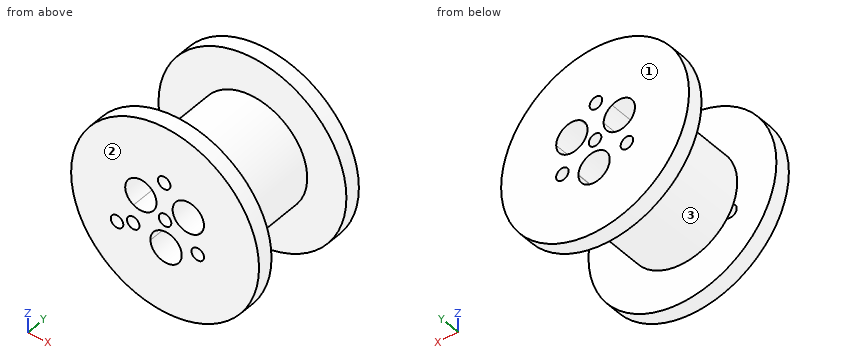
```python
from build123d import *

# Parameters (mm, degrees)
SKETCH1_R           = 30
BOSS_EXTRUDE1_DEPTH = 40
CUT_EXTRUDE1_START  = -5
SKETCH2_OUTSIDE_W   = 80.762
SKETCH2_OUTSIDE_H   = 80.762
SKETCH2_OUTSIDE_R   = 17.5
CUT_EXTRUDE1_DEPTH  = 30
SKETCH3_R           = 2
CUT_EXTRUDE2_DEPTH  = 59.309518948
CUT_EXTRUDE3_DEPTH  = 59.309518948
CUT_EXTRUDE4_REACH  = 57
SKETCH5_R           = 2
SKETCH8_R           = 2
CUT_EXTRUDE5_DEPTH  = 59.309518948


with BuildPart() as part:
    # Sketch1 → Boss-Extrude1 (new body)
    with BuildSketch(Plane(origin=(0, 0, 0), x_dir=(1, 0, 0), z_dir=(0, 1, 0))):
        with Locations(Location((0, 0, 0), (0, 0, 270))):
            Circle(SKETCH1_R)
    extrude(amount=BOSS_EXTRUDE1_DEPTH)

    # Sketch2 outside → Cut-Extrude1 (cut)
    with BuildSketch(Plane.XZ.offset(CUT_EXTRUDE1_START)):
        Rectangle(SKETCH2_OUTSIDE_W, SKETCH2_OUTSIDE_H)
        with Locations(Location((0, 0, 0), (0, 0, 270))):
            Circle(SKETCH2_OUTSIDE_R, mode=Mode.SUBTRACT)
    extrude(amount=-CUT_EXTRUDE1_DEPTH, mode=Mode.SUBTRACT)

    # Sketch3 → Cut-Extrude2 (cut, through all)
    with BuildSketch(Plane.XZ):
        with Locations(Location((0, 0, 0), (0, 0, 270))):
            Circle(SKETCH3_R)
    extrude(amount=-CUT_EXTRUDE2_DEPTH, mode=Mode.SUBTRACT)

    # Sketch4 → Cut-Extrude3 (cut, through all)
    with BuildSketch(Plane.XZ):
        with BuildLine():
            ThreePointArc((5.314601624, -8.562564428), (0.136244015, -3.747524192), (-4.678796221, -8.925881801))
            Line((-4.678796221, -8.925881801), (5.314601624, -8.562564428))
        make_face()
        with BuildLine():
            Line((5.314601624, -8.562564428), (-4.678796221, -8.925881801))
            ThreePointArc((-4.678796221, -8.925881801), (0.40874704, -13.743397777), (5.317902702, -8.744223114))
            ThreePointArc((5.317902702, -8.744223114), (5.317077364, -8.653378776), (5.314601624, -8.562564428))
        make_face()
        with BuildLine():
            ThreePointArc((4.758097504, 8.883862231), (3.177329144, 1.991752874), (10.069438501, 0.410984514))
            Line((10.069438501, 0.410984514), (4.758097504, 8.883862231))
        make_face()
        with BuildLine():
            Line((4.758097504, 8.883862231), (10.069438501, 0.410984514))
            ThreePointArc((10.069438501, 0.410984514), (11.788602428, 2.226509547), (12.413768003, 4.647423373))
            ThreePointArc((12.413768003, 4.647423373), (9.834681829, 9.022257798), (4.758097504, 8.883862231))
        make_face()
        with BuildLine():
            ThreePointArc((-5.39064228, 8.514897287), (-12.149768249, 6.437828165), (-10.072699128, -0.321297804))
            Line((-10.072699128, -0.321297804), (-5.39064228, 8.514897287))
        make_face()
        with BuildLine():
            Line((-5.39064228, 8.514897287), (-10.072699128, -0.321297804))
            ThreePointArc((-10.072699128, -0.321297804), (-5.153409868, -0.187190345), (-2.731670704, 4.096799742))
            ThreePointArc((-2.731670704, 4.096799742), (-3.447680618, 6.675060578), (-5.39064228, 8.514897287))
        make_face()
    extrude(amount=-CUT_EXTRUDE3_DEPTH, mode=Mode.SUBTRACT)

    # Sketch5 → Cut-Extrude4 (cut, up to next)
    with BuildSketch(Plane(origin=(0, 5, 0), x_dir=(1, 0, 0), z_dir=(0, 1, 0)), mode=Mode.PRIVATE) as cut_extrude4_sk1:
        with Locations(Location((-15.339737127, 8.422734999, 0), (0, 0, 270))):
            Circle(SKETCH5_R)
    cut_extrude4_tool1 = extrude(cut_extrude4_sk1.sketch, amount=-CUT_EXTRUDE4_REACH, mode=Mode.PRIVATE) & part.part
    add(cut_extrude4_tool1.solids().sort_by_distance((-15.339737, 5, -8.422735))[0], mode=Mode.SUBTRACT)

    # Sketch8 → Cut-Extrude5 (cut, through all)
    with BuildSketch(Plane(origin=(0, 40, 0), x_dir=(1, 0, 0), z_dir=(0, 1, 0))):
        with Locations(Location((-0.274503836, -11.904684903, 0), (0, 0, 270))):
            Circle(SKETCH8_R)
        with Locations(Location((10.446409645, 5.714285954, 0), (0, 0, 270))):
            Circle(SKETCH8_R)
        with Locations(Location((-10.172001933, 6.189762023, 0), (0, 0, 270))):
            Circle(SKETCH8_R)
    extrude(amount=-CUT_EXTRUDE5_DEPTH, mode=Mode.SUBTRACT)


solid = part.part
```
Can you work these out from the model? Positions are in its coordinate system, mm. Face numbers are marked on the shaded views. Round coordinates to 2 decimals unless told otherwise and drop trailing zeros. Loops run counter-clockwise (first coordinate to the right, second up) from the corner with the lowest first, then second, coordinate; pieces in that order, holes last.
Item 1: Suppose I cut it at B-B, the plane y = 23. Write out the boundary of the cut face in (x, z).
Item 2: Suppose I cut it at D-D, the plane y = 4. State how many separate pieces and enclosed holes the cut face has, then the cut area to 3 significant figures.
Item 3: Suppose I cut it at A-A, the plane x = -20.5. Write out the boundary of the cut face in (y, z).
Item 4: Please list where these lines run through material, in increasing order: L1, parallel to Y at x = 6.5, z = 26; L2, parallel to Z at x = -9, y = 29; L3, parallel to Z at x = -11, y = 18.
Item 5: Suppose I cut it at C-C, the plane x = 16. Write out the boundary of the cut face in (y, z).
Item 6: If we mould it in two halves opening along Y, with no side actions, what happens to the marked faces 1, 2 and 3? For each: +Y half, -Y half, draft (parallel to the pull), parting line (faces both ways), or undercut.
Item 7: Will these pins go through, and if not, where does the flat tip stop? pin 1 Ø12 at (y, z) = (10, -4) entering from -X; pin 2 Ø10 at (x, y) = (12, 28.5) entering from +Z; pin 3 Ø1 at (y, z) = (33, 22) entering from -X.
Reported:
1. outline: circle Ø35 at (0, 0); hole circle Ø10 at (-7.73, 4.1); hole circle Ø4 at (-10.17, -6.19); hole circle Ø4 at (-0.27, 11.9); hole circle Ø4 at (0, 0); hole circle Ø10 at (7.41, 4.65); hole (5.31, -8.56) arc R5 ccw (long way) to (5.32, -8.74) arc R5 ccw to start; hole circle Ø4 at (10.45, -5.71)
2. separate pieces: 1
2. enclosed holes: 8
2. area: 2,530 mm2
3. outline: (0, -21.9) - (5, -21.9) - (5, 21.9) - (0, 21.9) - close; (35, -21.9) - (40, -21.9) - (40, 21.9) - (35, 21.9) - close
4. L1: y = 0 to 5, 35 to 40
4. L2: z = -15.01 to -7.81, -4.57 to -0.74, 8.93 to 15.01
4. L3: z = -13.61 to -8.01, -4.37 to 0.31, 7.88 to 13.61
5. outline: (0, -25.38) - (5, -25.38) - (5, -7.09) - (35, -7.09) - (35, -25.38) - (40, -25.38) - (40, 25.38) - (35, 25.38) - (35, 7.09) - (5, 7.09) - (5, 25.38) - (0, 25.38) - close
6. face 1: +Y half
6. face 2: -Y half
6. face 3: undercut
7. pin 1: stops at x = -29.99
7. pin 2: stops at z = 16.04
7. pin 3: passes through
